from build123d import *

# Parameters (mm, degrees)
SKETCH_1_R          = 17.5
EXTRUDE_1_DEPTH     = 30
SKETCH_2_R          = 20
EXTRUDE_2_DEPTH     = 25
EXTRUDE_5_DEPTH     = 2
SKETCH_7_W          = 2
SKETCH_7_H          = 45
EXTRUDE_6_DEPTH     = 45
FILLET_3_R          = 5
SKETCH_8_R          = 1.5
CUT_EXTRUDE_1_DEPTH = 5
SKETCH_9_R          = 15
CUT_EXTRUDE_2_DEPTH = 10
EXTRUDE_7_DEPTH     = 70
SKETCH_11_R         = 1.5
CUT_EXTRUDE_3_DEPTH = 2


with BuildPart() as part:
    # 草图1 → 凸台-拉伸1 (new body)
    with BuildSketch(Plane.XY):
        Circle(SKETCH_1_R)
    extrude(amount=EXTRUDE_1_DEPTH)

    # 草图2 → 凸台-拉伸2 (add)
    with BuildSketch(Plane.XY.offset(30)):
        Circle(SKETCH_2_R)
    extrude(amount=EXTRUDE_2_DEPTH)

    # 草图6 → 凸台-拉伸5 (add)
    with BuildSketch(Plane.XY.offset(55)):
        with BuildLine():
            Line((0, 22.5), (-35, 22.5))
            Line((-35, 22.5), (-35, -22.5))
            Line((-35, -22.5), (0, -22.5))
            ThreePointArc((0, -22.5), (22.5, 0), (0, 22.5))
        make_face()
    extrude(amount=EXTRUDE_5_DEPTH)

    # 草图7 → 凸台-拉伸6 (add)
    with BuildSketch(Plane.XY.offset(57)):
        with Locations((-34, 0)):
            Rectangle(SKETCH_7_W, SKETCH_7_H)
    extrude(amount=-EXTRUDE_6_DEPTH)

    # 圆角3
    fillet_3_edges = [part.edges().sort_by_distance(p)[0] for p in [
        (-35, 0, 57),
        (-33, 0, 55),
    ]]
    fillet(fillet_3_edges, radius=FILLET_3_R)

    # 草图8 → 切除-拉伸1 (cut)
    with BuildSketch(Plane.ZY.offset(35)):
        with Locations((22, 15)):
            Circle(SKETCH_8_R)
        with Locations((22, -15)):
            Circle(SKETCH_8_R)
        with Locations((46, 15)):
            Circle(SKETCH_8_R)
        with Locations((46, -15)):
            Circle(SKETCH_8_R)
    extrude(amount=-CUT_EXTRUDE_1_DEPTH, mode=Mode.SUBTRACT)

    # 草图9 → 切除-拉伸2 (cut)
    with BuildSketch(Plane(origin=(0, 0, 55), x_dir=(-1, 0, 0), z_dir=(0, 0, -1))):
        Circle(SKETCH_9_R)
    extrude(amount=-CUT_EXTRUDE_2_DEPTH, mode=Mode.SUBTRACT)

    # 草图10 → 凸台-拉伸7 (add)
    with BuildSketch(Plane(origin=(0, 0, 0), x_dir=(-1, 0, 0), z_dir=(0, 0, -1))):
        with BuildLine():
            Line((6.4409075, 3.842487551), (6.4409075, -3.842487551))
            ThreePointArc((6.4409075, -3.842487551), (-7.5, 0), (6.4409075, 3.842487551))
        make_face()
    extrude(amount=-EXTRUDE_7_DEPTH)

    # 草图11 → 切除-拉伸3 (cut)
    with BuildSketch(Plane.XY.offset(57)):
        with Locations((0, 18.605053308)):
            Circle(SKETCH_11_R)
        with Locations((16.112448804, 9.302526654)):
            Circle(SKETCH_11_R)
        with Locations((16.112448804, -9.302526654)):
            Circle(SKETCH_11_R)
        with Locations((0, -18.605053308)):
            Circle(SKETCH_11_R)
        with Locations((-16.112448804, -9.302526654)):
            Circle(SKETCH_11_R)
        with Locations((-16.112448804, 9.302526654)):
            Circle(SKETCH_11_R)
    extrude(amount=-CUT_EXTRUDE_3_DEPTH, mode=Mode.SUBTRACT)


solid = part.part
Model file for the job. Use its own axes, mm. A direction names the side the tool comes from. Round coordinates to 2 decimals unless told otherwise and drop trailing zeros. Loops run counter-clockwise (first coordinate to the right, second up) from the corner with the lowest first, then second, coordinate; pieces in that order, holes last. Notation, with made-up numbers: (-17.5, 59.25) - (15.5, 59.25) arc R15 ccw to (15.5, 64.25) - close; hole circle Ø10 at (84, 25). An arc over 180 degrees is marked (long way). Write each question's results on one line, items separated by ' | '.
(1) Saw through at A-A, the plane z = 22. List the corners of the cut face in (x, y).
Answer below:
outline: (-35, -22.5) - (-33, -22.5) - (-33, -16.5) - (-35, -16.5) - close; (-35, -13.5) - (-33, -13.5) - (-33, 13.5) - (-35, 13.5) - close; (-35, 16.5) - (-33, 16.5) - (-33, 22.5) - (-35, 22.5) - close; circle Ø35 at (0, 0)
(2) Mould opens along X. For faces 1 (the cylindrical face through (-34, 0, 55)), 2 (the cylindrical face through (15.007, -8.289, 56.014)), 3 (the flat face through (0, 0, 0)) say: released by +X, released by -X, zero draft, split by the parting line, or undercut.
Answer below:
face 1: released by -X | face 2: undercut | face 3: zero draft
(3) Saw through at B-B, the plane y = 0. List the corners of the cut face in (x, z).
Answer below:
outline: (-35, 12) - (-33, 12) - (-33, 50) arc R5 cw to (-28, 55) - (-20, 55) - (-20, 30) - (-17.5, 30) - (-17.5, 0) - (17.5, 0) - (17.5, 30) - (20, 30) - (20, 55) - (22.5, 55) - (22.5, 57) - (15, 57) - (15, 55) - (7.5, 55) - (7.5, 70) - (-6.44, 70) - (-6.44, 55) - (-15, 55) - (-15, 57) - (-30, 57) arc R5 ccw to (-35, 52) - close
(4) 3-axis set-ups, long thin cutter, end or side, ignore diameter. For faces 4 (the cylindrical face through (-34.01, 15.07, 44.5)), 5 (the flat face through (-35, 0, 32)), 6 (the flat face through (-34, 0, 12)), 7 (the cylindrical face through (7.495, -0.273, 62.395)): which of +Z, -Z, +X, -X, +Y, -Y reach the whole face in a straight line?
Answer below:
face 4: -X | face 5: +Z, -Z, -X, +Y, -Y | face 6: -Z, -X, +Y, -Y | face 7: +Z
(5) Saw through at D-D, the plane x = -23. List the corners of the cut face in (y, z), then the cut area to 3 significant figures.
Answer below:
outline: (-22.5, 55) - (22.5, 55) - (22.5, 57) - (-22.5, 57) - close | area: 90.0 mm^2
(6) Pin check, flat tips, straight feed: pin 1 (3 mm diameter, centred on x = -19.5, y = -8.5, fed in from +Z); pin 2 (0.6 mm diameter, centred on x = -34.5, y = 4.5, fed in from -Z); pin 3 (2.5 mm diameter, centred on x = 16.11, y = 9.3, fed in from +Z). Stop position of each tip, or through.
Answer below:
pin 1: stops at z = 57 | pin 2: stops at z = 12 | pin 3: stops at z = 55
(7) Wall check: L1, parallel to Y at x = -34.2, z = 22; L2, parallel to Z at x = -9.5, y = -3; L3, parallel to X at y = 6.5, z = 17.5. Give the ranges that are in metal, low to high.
Answer below:
L1: y = -22.5 to -16.5, -13.5 to 13.5, 16.5 to 22.5 | L2: z = 0 to 55 | L3: x = -35 to -33, -16.25 to 16.25
(8) Saw through at C-C, the plane z = 49. List the corners of the cut face in (x, y).
Answer below:
outline: (-35, -22.5) - (-33, -22.5) - (-33, 22.5) - (-35, 22.5) - close; circle Ø40 at (0, 0)
